from build123d import *

# Parameters (mm, degrees)
BOSS_EXTRUDE1_DEPTH     = 50
CUT_EXTRUDE1_DEPTH      = 68.292354146
CUT_EXTRUDE1_DEPTH_BACK = 68.292354146
SKETCH3_R               = 1.75
BOSS_EXTRUDE2_DEPTH     = 0.1
BOSS_EXTRUDE3_START     = 0.5
SKETCH5_R               = 1.75
BOSS_EXTRUDE3_DEPTH     = 0.5
SKETCH4_R               = 1.1
CUT_EXTRUDE2_DEPTH      = 61.952851438
BOSS_EXTRUDE4_REACH     = 62.971
BOSS_EXTRUDE5_START     = 2
BOSS_EXTRUDE5_DEPTH     = 2
SKETCH8_R               = 0.625
CUT_EXTRUDE3_DEPTH      = 65.090580501


with BuildPart() as part:
    # Sketch1 → Boss-Extrude1 (new body)
    with BuildSketch(Plane.XY):
        with BuildLine():
            Line((-15, 0), (44.999916667, 0))
            Line((44.999916667, 0), (44.999916667, 0.1))
            add(Edge.make_bspline(
                [(-15, 0), (-15, 3.230995927), (19.077066257, 1.403070244), (44.999916667, 0.1)],
                knots=[0, 0, 0, 0, 1, 1, 1, 1], degree=3))
        make_face()
    boss_extrude1 = extrude(amount=BOSS_EXTRUDE1_DEPTH)

    # Mirror1: Boss-Extrude1 across plane
    add(boss_extrude1.mirror(Plane(origin=(-15, 0, 50), x_dir=(0, 0, 1), z_dir=(0, 1, 0))))

    # Sketch2 → Cut-Extrude1 (cut, two sides: drawn at the far end of the back side and taken through both)
    with BuildSketch(Plane(origin=(0, 0, 0), x_dir=(1, 0, 0), z_dir=(0, 1, 0)).offset(-CUT_EXTRUDE1_DEPTH_BACK)):
        Polygon((-26.522782457, -38.79799257), (-2.5, -50), (2.5, -50), (51.792235583, -27.01465306), (51.792235583, -55.115877471), (-26.522782457, -55.115877471), align=None)
        Polygon((-2.5, -15), (2.5, -15), (50.354863493, -8.27443754), (50.354863493, 7.109448332), (-22.823153077, 7.109448332), (-22.823153077, -15), align=None)
    extrude(amount=CUT_EXTRUDE1_DEPTH + CUT_EXTRUDE1_DEPTH_BACK, mode=Mode.SUBTRACT)

    # Sketch3 → Boss-Extrude2 (add)
    with BuildSketch(Plane.XY.offset(50)):
        Circle(SKETCH3_R)
    extrude(amount=BOSS_EXTRUDE2_DEPTH)

    # Sketch5 → Boss-Extrude3 (add)
    with BuildSketch(Plane(origin=(0, 0, 15), x_dir=(-1, 0, 0), z_dir=(0, 0, -1)).offset(BOSS_EXTRUDE3_START)):
        with Locations(Location((0, 0, 0), (0, 0, 180))):
            Circle(SKETCH5_R)
    extrude(amount=-BOSS_EXTRUDE3_DEPTH)

    # Sketch4 → Cut-Extrude2 (cut, through all)
    with BuildSketch(Plane.XY.offset(50.1)):
        Circle(SKETCH4_R)
    extrude(amount=-CUT_EXTRUDE2_DEPTH, mode=Mode.SUBTRACT)

    # Boss-Extrude4: up to this plane
    boss_extrude4_end = Plane(origin=(50.354863493, -1.966265525, 8.27443754), z_dir=(0.13917310096005872, 0, 0.9902680687415713))
    # Sketch6 → Boss-Extrude4 (add, up to the surface)
    with BuildSketch(Plane(origin=(0, 0, 9), x_dir=(-1, 0, 0), z_dir=(0, 0, -1)), mode=Mode.PRIVATE) as boss_extrude4_sk1:
        with BuildLine():
            Line((-6, -1.375), (-14, -1.375))
            ThreePointArc((-14, -1.375), (-15.375, 0), (-14, 1.375))
            Line((-14, 1.375), (-6, 1.375))
            ThreePointArc((-6, 1.375), (-4.625, 0), (-6, -1.375))
        make_face()
    boss_extrude4_tool1 = split(extrude(boss_extrude4_sk1.sketch, amount=-BOSS_EXTRUDE4_REACH, mode=Mode.PRIVATE), bisect_by=boss_extrude4_end, keep=Keep.BOTH, mode=Mode.PRIVATE)
    add(boss_extrude4_tool1.solids().sort_by_distance((10, 0, 9))[0])

    # Sketch7 → Boss-Extrude5 (add)
    with BuildSketch(Plane(origin=(0, 0, 9), x_dir=(-1, 0, 0), z_dir=(0, 0, -1)).offset(BOSS_EXTRUDE5_START)):
        with BuildLine():
            Line((-4.853696051, -0.759349891), (2.501026797, 10.343236601))
            ThreePointArc((2.501026797, 10.343236601), (1.885205071, 14.333667037), (-2.145513036, 14.096848543))
            Line((-2.145513036, 14.096848543), (-14.983360142, 0.961055582))
            ThreePointArc((-14.983360142, 0.961055582), (-15.26729563, -0.533466763), (-14, -1.375))
            Line((-14, -1.375), (-6, -1.375))
            ThreePointArc((-6, -1.375), (-5.34941607, -1.211348649), (-4.853696051, -0.759349891))
        make_face()
    extrude(amount=-BOSS_EXTRUDE5_DEPTH)

    # Sketch8 → Cut-Extrude3 (cut, through all)
    with BuildSketch(Plane(origin=(0, 0, 7), x_dir=(-1, 0, 0), z_dir=(0, 0, -1))):
        with Locations((0, 12)):
            Circle(SKETCH8_R)
    extrude(amount=-CUT_EXTRUDE3_DEPTH, mode=Mode.SUBTRACT)


solid = part.part
Source: CAD feature listing. Evaluate the final solid. Frame: model axes, mm. A direction names the side the tool comes from. Round coordinates to 2 decimals unless told otherwise and drop trailing zeros. Write each loop counter-clockwise with the first axis right and the second up, starting at its lowest first coordinate (ties: lowest second). Pieces come first, ordered by that corner, then holes. Notation, with made-up numbers: M -9,-40 L 4,-40 A29 cw 4,-19 Z; hole C 86,-30 d6. An arc over 180 degrees is marked long. One line per item, written item: value. Start each with the question number.
Item 1: Section query D-D (y = 9). Return the cut outline in (x, z).
Item 2: Mould query, pull axis X, two halves, no side actions, for faces 6 (the cylindrical face through (1.617, 0.67, 14.746)), 7 (the flat face through (-7.45, -0.03, 47.69)), 8 (the flat face through (-1, 1, 14.5)), 9 (the cylindrical face through (-1.933, 14.294, 7.986)). Classes: pulls with the +X half, pulls with the -X half, needs draft (parallel to the pull), parting line crosses it, or undercut.
Item 3: Section query A-A (y = 12). Return the cut outline in (x, z) (3 decimals), plus the area to 3 significant figures.
Item 4: Pin query (flat end, axial travel): pin 1 (12 mm diameter, centred on x = 19.5, z = 14, fed in from +Y); pin 2 (1.7 mm diameter, centred on x = 10, z = 11, fed in from +Y) (3 decimals); pin 3 (8 mm diameter, centred on x = 4, y = 6, fed in from +Z). Return the tip coordinate at first contact, or that it passes through.
Item 5: Section query C-C (y = 5.75). Return the cut outline in (x, z).
Item 6: Section query B-B (x = 0). State how many separate pieces and enclosed holes the cut face has, plus the area to 3 significant figures.
Item 7: Ray query, L1, parallel to Y at x = 0, z = 28; L2, parallel to X at y = 0.25, z = 36; L3, parallel to Y at x = 0, z = 8 (3 decimals). Return the intervals inside material, ascending. Write a range as from..to.
Item 8: Set-up query: faces 1 (the cylindrical face through (1.05, 0.33, 32.55)), 2 (the flat face through (10, 1.375, 12)), 3 (the flat face through (-2, 0, 50)), 4 (the flat face through (1.23, 4.71, 7.99)), 5 (the flat face through (-1, -1, 50.1)). Return all of +Z, -Z, +X, -X, +Y, -Y with unobstructed straight access to the full face (end or side cutting, diameter ignored); none if empty.
Result set:
1. outline: M -1.61,7 L 7.13,7 L 7.13,9 L -1.61,9 Z
2. face 6: undercut
2. face 7: pulls with the -X half
2. face 8: needs draft
2. face 9: parting line crosses it
3. outline: M -3,7 L -0.625,7 L -0.625,9 L -3,9 Z; M 0.625,7 L 4.195,7 L 4.195,9 L 0.625,9 Z
3. area: 11.9 mm²
4. pin 1: stops at y = 1.53
4. pin 2: stops at y = 1.375
4. pin 3: stops at z = 9
5. outline: M 0.54,7 L 10.3,7 L 10.3,9 L 0.54,9 Z
6. separate pieces: 4
6. enclosed holes: 0
6. area: 64.7 mm²
7. L1: y = -1.81..-1.1, 1.1..1.81
7. L2: x = -14.93..-1.07, 1.07..32.52
7. L3: y = 6.568..11.375, 12.625..15
8. face 1: +Z, -Z
8. face 2: -X, +Y
8. face 3: +Z
8. face 4: -Z, -X, -Y
8. face 5: +Z, +X, -X, +Y, -Y
